```python
from build123d import *

# Parameters (mm, degrees)
SKETCH_1_R      = 1.525
EXTRUDE_1_DEPTH = 5
EXTRUDE_START   = -4
EXTRUDE_4_DEPTH = 4
FILLET_1_R      = 2
FILLET_2_R      = 5
FILLET_3_R      = 2


with BuildPart() as part:
    # 草图1 → 凸台-拉伸1 (new body)
    with BuildSketch(Plane(origin=(0, 0, 0), x_dir=(1, 0, 0), z_dir=(0, 1, 0))):
        with BuildLine():
            Line((3.9, -3.732227301), (3.9, 2.55))
            Line((3.9, 2.55), (5.747877547, 2.55))
            Line((5.747877547, 2.55), (8.9, 2.55))
            Line((8.9, 2.55), (8.9, 13.6))
            Line((8.9, 13.6), (3.9, 13.6))
            Line((3.9, 13.6), (3.9, 13.765734151))
            Line((3.9, 13.765734151), (3.9, 26))
            ThreePointArc((3.9, 26), (3.021320344, 28.121320344), (0.9, 29))
            Line((0.9, 29), (-0.9, 29))
            ThreePointArc((-0.9, 29), (-3.021320344, 28.121320344), (-3.9, 26))
            Line((-3.9, 26), (-3.9, 8.75))
            Line((-3.9, 8.75), (-4.851185593, 8.773222699))
            ThreePointArc((-4.851185593, 8.773222699), (-6.29684845, 8.205186518), (-6.9, 6.773818499))
            Line((-6.9, 6.773818499), (-6.9, 3.9))
            Line((-6.9, 3.9), (-15.75, 3.9))
            ThreePointArc((-15.75, 3.9), (-17.871320344, 3.021320344), (-18.75, 0.9))
            Line((-18.75, 0.9), (-18.75, -0.9))
            ThreePointArc((-18.75, -0.9), (-17.871320344, -3.021320344), (-15.75, -3.9))
            Line((-15.75, -3.9), (0, -3.9))
            Line((0, -3.9), (3.9, -3.9))
            Line((3.9, -3.9), (3.9, -3.732227301))
        make_face()
        with Locations(Location((0, 0, 0), (0, 0, 270))):
            Circle(SKETCH_1_R, mode=Mode.SUBTRACT)
    extrude(amount=EXTRUDE_1_DEPTH)

    # 草图4 → 凸台-拉伸4 (add)
    with BuildSketch(Plane(origin=(0, 0, 0), x_dir=(1, 0, 0), z_dir=(0, 1, 0)).offset(EXTRUDE_START)):
        with BuildLine():
            Line((-6.9, 3.9), (-3.9, 3.9))
            Line((-3.9, 3.9), (-3.9, 8.75))
            Line((-3.9, 8.75), (-4.851185593, 8.773222699))
            ThreePointArc((-4.851185593, 8.773222699), (-6.29684845, 8.205186518), (-6.9, 6.773818499))
            Line((-6.9, 6.773818499), (-6.9, 3.9))
        make_face()
    extrude(amount=EXTRUDE_4_DEPTH)

    # 圆角1
    fillet_1_edges = [part.edges().sort_by_distance(p)[0] for p in [
        (3.9, 2.5, 3.9),
    ]]
    fillet(fillet_1_edges, radius=FILLET_1_R)

    # 圆角2
    fillet_2_edges = [part.edges().sort_by_distance(p)[0] for p in [
        (8.9, 2.5, -13.6),
    ]]
    fillet(fillet_2_edges, radius=FILLET_2_R - 0.0001)  # a hair under: the kernel refuses the full size

    # 圆角3
    fillet_3_edges = [part.edges().sort_by_distance(p)[0] for p in [
        (3.9, 2.5, -2.55),
    ]]
    fillet(fillet_3_edges, radius=FILLET_3_R)


solid = part.part
```
The listing builds one solid part. Answer for the finished solid, in the listing's coordinates (mm). A direction names the side the tool comes from. Coordinates: 2 decimals unless noted, no trailing zeros. Loops run counter-clockwise (first coordinate to the right, second up) from the corner with the lowest first, then second, coordinate; pieces in that order, holes last. Notation, with made-up numbers: (59.5, 43.5) - (94.5, 43.5) arc R12 ccw to (94.5, 61.5) - close; hole circle Ø9 at (72.25, -1.75). An arc over 180 degrees is marked (long way). Write item = value, one per line.
1) Section D-D (z = -6) is taken. Determine the outline of the cut face in (x, y).
Responses:
outline = (-6.9, -4) - (-3.9, -4) - (-3.9, 0) - (8.9, 0) - (8.9, 5) - (-6.9, 5) - close
2) Section B-B (x = 0) is taken. Determine the outline of the cut face in (y, z) (3 decimals).
Responses:
outline = (0, -29) - (5, -29) - (5, -1.525) - (0, -1.525) - close; (0, 1.525) - (5, 1.525) - (5, 3.9) - (0, 3.9) - close
3) Determine the mould class of faces 1 (the face through (-17.85, 2.46, -3.04)), 2 (the face through (7, 2, -2.55)), 3 (the face through (8.9, 2, -6)) for opening direction X: pulls with the +X half, pulls with the -X half, needs draft (parallel to the pull), parting line crosses it, or undercut.
Responses:
face_1 = pulls with the -X half
face_2 = needs draft
face_3 = pulls with the +X half
4) Each of these flat-tipped pins is pushed along its axis until it touches: P1, Ø0.7, axis at y = 2, z = 0.5, coming from the +X side; P2, Ø4, axis at x = -10.5, y = 3, coming from the -Z side; P3, Ø0.9, axis at x = 8, y = 2, coming from the +Z side; P4, Ø10, axis at x = -10.5, z = -21.5, coming from the +Y side. Where does it stop, or does it pass through?
Responses:
P1 = 3.9
P2 = -3.9
P3 = -2.55
P4 = through
5) Section A-A (z = 0) is taken. Determine the outline of the cut face in (x, y) (3 decimals).
Responses:
outline = (-18.75, 0) - (-1.525, 0) - (-1.525, 5) - (-18.75, 5) - close; (1.525, 0) - (3.9, 0) - (3.9, 5) - (1.525, 5) - close
6) Which of the six approach directions +Z, -Z, +X, -X, +Y, -Y give full straight-line access (tool end or side, diameter ignored) to faces 4 (the face through (3.9, 2, -20)), 5 (the face through (-3.9, -2, -6)), 6 (the face through (3.9, 2, 1)), 7 (the face through (-5, -2, -3.9))?
Responses:
face_4 = -Z, +X, +Y, -Y
face_5 = +Z, -Z, +X, -Y
face_6 = +Z, +X, +Y, -Y
face_7 = +Z, +X, -X, -Y
7) Find the intervals of material crossed by line 1 along X through (y, z) = (1.05, 0) (3 decimals); line 2 along Y through (x, z) = (2.25, -12); line 3 along Z through (x, y) = (-9.75, 3.5), in increasing order.
Responses:
line_1 = -18.75 to -1.525, 1.525 to 3.9
line_2 = 0 to 5
line_3 = -3.9 to 3.9
